Autodesk Fusion 360 part; units mm, degrees
sketch "スケッチ1" plane through (0, 0, 0) normal (0, 0, 1) x (1, 0, 0)
  arc A0 (20.7798, 184.0311) -> (8, 170.0843) centre (22, 170.0843) ccw
  line L0 (90, 190.087) -> (20.7798, 184.0311)
  line L1 (0, 200) -> (0, 0)
  line L2 (8, 170.0843) -> (8, 29.9157)
  line L3 (0, 0) -> (90, 0)
  line L4 (20.7798, 15.9689) -> (90, 9.913)
  arc A1 (8, 29.9157) -> (20.7798, 15.9689) centre (22, 29.9157) ccw
  line L5 (90, 9.913) -> (90, 0)
  line L6 (0, 200) -> (90, 200)
  line L7 (90, 200) -> (90, 190.087)
extrude "押し出し1" add sketch "スケッチ1" along normal blind 100
Check sheet for the modelled part. Datum: model origin and axes. Units: mm. A direction names the side the tool comes from. Round coordinates to 2 decimals unless told otherwise and drop trailing zeros. Order: outer loops, then holes, each group sorted by start corner. A loop starts at its lowest first (then second) coordinate and runs counter-clockwise, first axis right, second up. Notation, with made-up numbers: (48, 58.25) - (94, 58.25) arc R34 ccw to (94, 92.25) - close; hole circle Ø3 at (80.25, 53). An arc over 180 degrees is marked (long way). Write item = value, one per line.
Q1. Section check B-B (z = 42). Record the boundary of the cut face in (x, y), and give its area (3 significant figures).
Computed:
outline = (0, 0) - (90, 0) - (90, 9.91) - (20.78, 15.97) arc R14 cw to (8, 29.92) - (8, 170.08) arc R14 cw to (20.78, 184.03) - (90, 190.09) - (90, 200) - (0, 200) - close
area = 3,880 mm^2
Q2. Tool access check on faces 4 (the face through (55.87, 187.1, 49.3)), 5 (the face through (5, 100, 100)). Record the directions out of +Z, -Z, +X, -X, +Y, -Y that give a thin tool (end or side, any length) a straight path to the whole face; none if there is none.
Computed:
face_4 = +Z, -Z, +X
face_5 = +Z, +X, -X, +Y, -Y
Q3. Section check D-D (y = 130.5). Record the boundary of the cut face in (x, z), and give its area (3 significant figures).
Computed:
outline = (0, 0) - (8, 0) - (8, 100) - (0, 100) - close
area = 800 mm^2
Q4. Go/stop test with flat-tipped pins: pin 1 (2 mm diameter, centred on x = 32, z = 63, fed in from -Y); pin 2 (4 mm diameter, centred on x = 11.5, y = 47.5, fed in from +Z). Record where each tip stops, or that it passes through.
Computed:
pin_1 = 0
pin_2 = through
Q5. Thickness scan on line 1 along X through (y, z) = (99, 79); line 2 along Y through (x, z) = (37, 33.5); line 3 along Y through (x, z) = (33.5, 87). Record the ranges inside material, lowest first.
Computed:
line_1 = 0 to 8
line_2 = 0 to 14.55, 185.45 to 200
line_3 = 0 to 14.86, 185.14 to 200
Q6. Section check C-C (x = 81). Record the boundary of the cut face in (y, z), and give its area (3 significant figures).
Computed:
outline = (0, 0) - (10.7, 0) - (10.7, 100) - (0, 100) - close; (189.3, 0) - (200, 0) - (200, 100) - (189.3, 100) - close
area = 2,140 mm^2
Q7. Draft check along Y on faces 1 (the face through (44, 0, 49)), 2 (the face through (0, 101, 49)), 3 (the face through (54.905, 12.983, 49.3)). Enter one of: pulls with the +Y half, pulls with the -Y half, needs draft (parallel to the pull), parting line crosses it, or undercut.
Computed:
face_1 = pulls with the -Y half
face_2 = needs draft
face_3 = undercut
Q8. Section check A-A (x = 42.5). Record the boundary of the cut face in (y, z), and give its area (3 significant figures).
Computed:
outline = (0, 0) - (14.07, 0) - (14.07, 100) - (0, 100) - close; (185.93, 0) - (200, 0) - (200, 100) - (185.93, 100) - close
area = 2,810 mm^2
